```python
from build123d import *

# Parameters (mm, degrees)
BOSS_EXTRUDE1_DEPTH         = 3
SKETCH2_W                   = 20.0076
SKETCH2_H                   = 4.999999987
BOSS_EXTRUDE2_DEPTH         = 8
BOSS_EXTRUDE3_DEPTH         = 8
SKETCH4_W                   = 12.0076
SKETCH4_H                   = 1.4
CUT_EXTRUDE1_DEPTH          = 27.7
TAP_DRILL_FOR_M3_TAP1_D     = 2.5
TAP_DRILL_FOR_M3_TAP1_DEPTH = 15.5
TAP_DRILL_FOR_M3_TAP1_TIP   = 0.751075774


with BuildPart() as part:
    # Sketch1 → Boss-Extrude1 (new body)
    with BuildSketch(Plane.XY):
        Polygon((24.618539046, -84.902707764), (24.618539046, -85.849818272), (20.618539046, -85.849818272), (20.618539046, -73.202707764), (40.626139046, -73.202707764), (40.626139046, -85.849818272), (36.626139046, -85.849818272), (36.626139046, -84.902707764), align=None)
    extrude(amount=BOSS_EXTRUDE1_DEPTH)

    # Sketch2 → Boss-Extrude2 (add)
    with BuildSketch(Plane(origin=(0, 0, 0), x_dir=(-1, 0, 0), z_dir=(0, 0, -1))):
        with Locations((-30.622339046, -75.702707758)):
            Rectangle(SKETCH2_W, SKETCH2_H)
    extrude(amount=BOSS_EXTRUDE2_DEPTH)

    # Sketch3 → Boss-Extrude3 (add)
    with BuildSketch(Plane(origin=(0, 0, 0), x_dir=(-1, 0, 0), z_dir=(0, 0, -1))):
        Polygon((-40.626139046, -82.202707751), (-40.626139046, -85.849818272), (-36.626139046, -85.849818272), (-36.626139046, -84.902707764), (-24.618539046, -84.902707764), (-24.618539046, -85.849818272), (-20.618539046, -85.849818272), (-20.618539046, -82.202707751), align=None)
    extrude(amount=BOSS_EXTRUDE3_DEPTH)

    # Sketch4 → Cut-Extrude1 (cut)
    with BuildSketch(Plane.XY.offset(3)):
        with Locations((30.622339046, -73.902707764)):
            Rectangle(SKETCH4_W, SKETCH4_H)
    extrude(amount=-CUT_EXTRUDE1_DEPTH, mode=Mode.SUBTRACT)

    # Tap Drill for M3 Tap1
    with Locations(Plane(origin=(0, -73.202707764, 0), x_dir=(1, 0, 0), z_dir=(0, 1, 0))):
        with Locations((22.618539046, 6), (38.626139046, 6)):
            Hole(TAP_DRILL_FOR_M3_TAP1_D / 2, depth=TAP_DRILL_FOR_M3_TAP1_DEPTH)
            with Locations((0, 0, -(TAP_DRILL_FOR_M3_TAP1_DEPTH + TAP_DRILL_FOR_M3_TAP1_TIP / 2))):  # 118° drill point
                Cone(0, TAP_DRILL_FOR_M3_TAP1_D / 2, TAP_DRILL_FOR_M3_TAP1_TIP, mode=Mode.SUBTRACT)


solid = part.part
```
The listing builds one solid part. Answer for the finished solid, in the listing's coordinates (mm). A direction names the side the tool comes from. Coordinates: 2 decimals unless noted, no trailing zeros. Order: outer loops, then holes, each group sorted by start corner. A loop starts at its lowest first (then second) coordinate and runs counter-clockwise, first axis right, second up. Notation, with made-up numbers: M 83,47.25 L 116,47.25 A20 ccw 116,86.25 Z; hole C -7,-24.5 d4. An arc over 180 degrees is marked long. Answer as a JSON object with one key per item and string values. Group by question number.
1. Section B-B on z = -6 is taken. State how many separate pieces and enclosed holes the cut face has, then the cut area to 3 significant figures.
2. A tool of negligible diameter and unlimited length cuts with its end or side. For faces 1 (the flat face through (24.619, -85.4, -2.4)), 2 (the flat face through (24.619, -74, -2)), 3 (the flat face through (31, -76, -8)), from which of +Z, -Z, +X, -X, +Y, -Y can it reach the whole face along a straight path? Write none if from no direction.
3. Flat-ended cylindrical pins translate along their axes: P1, Ø3, axis at y = -80.5, z = -3.5, coming from the -X side (3 decimals); P2, Ø3, axis at x = 22.62, z = -6, coming from the -Y side; P3, Ø3, axis at x = 31, z = -0.5, coming from the +Y side; P4, Ø1.2, axis at x = 33, y = -80, coming from the -Z side. Find the tip coordinate at first contact, or state that the pin passes through.
4. Section C-C on x = 23.5 is taken. Write down the section's boundary in (y, z), then the cut area to 3 significant figures.
5. Section A-A on z = -3 is taken. Write down the section's boundary in (x, y).
6. Straight lines are drawn through the part: line 1 (X direction, y = -74.75, z = -6); line 2 (Y direction, x = 33, z = -4); line 3 (Y direction, x = 37.5, z = -1.75). For each, find the intervals that lie inside material, in ascending order.
7. Section D-D on y = -76.75 is taken. Write down the section's boundary in (x, z), then the cut area to 3 significant figures.
8. Determine the mould class of faces 4 (the flat face through (31, -84.903, -2)), 5 (the flat face through (30, -82.203, -4)), 6 (the flat face through (31, -78.203, -4)), 7 (the cylindrical face through (22.89, -84.05, -4.78)) for opening direction Y: released by +Y, released by -Y, zero draft, split by the parting line, or undercut.
Values follow:
{
 "1": {"separate pieces": "6", "enclosed holes": "0", "area": "102 mm2"},
 "2": {"face 1": "+Z, -Z, -Y", "face 2": "+Z, -Z, +Y", "face 3": "-Z, +X, -X, +Y, -Y"},
 "3": {"P1": "through", "P2": "y = -85.85", "P3": "y = -74.6", "P4": "z = 0"},
 "4": {"outline": "M -85.85,-8 L -82.2,-8 L -82.2,-6.89 L -85.85,-6.89 Z; M -85.85,-5.11 L -82.2,-5.11 L -82.2,0 L -78.2,0 L -78.2,-5.11 L -73.2,-5.11 L -73.2,3 L -85.85,3 Z; M -78.2,-8 L -73.2,-8 L -73.2,-6.89 L -78.2,-6.89 Z", "area": "91.8 mm2"},
 "5": {"outline": "M 20.62,-85.85 L 24.62,-85.85 L 24.62,-84.9 L 36.63,-84.9 L 36.63,-85.85 L 40.63,-85.85 L 40.63,-82.2 L 20.62,-82.2 Z; M 20.62,-78.2 L 40.63,-78.2 L 40.63,-73.2 L 36.63,-73.2 L 36.63,-74.6 L 24.62,-74.6 L 24.62,-73.2 L 20.62,-73.2 Z"},
 "6": {"line 1": "20.62 to 21.37, 23.87 to 37.38, 39.88 to 40.63", "line 2": "-84.9 to -82.2, -78.2 to -74.6", "line 3": "-85.85 to -82.2, -78.2 to -73.2"},
 "7": {"outline": "M 20.62,-8 L 40.63,-8 L 40.63,3 L 20.62,3 Z; hole C 22.62,-6 d2.5; hole C 38.63,-6 d2.5", "area": "210 mm2"},
 "8": {"face 4": "released by -Y", "face 5": "undercut", "face 6": "undercut", "face 7": "zero draft"}
}
